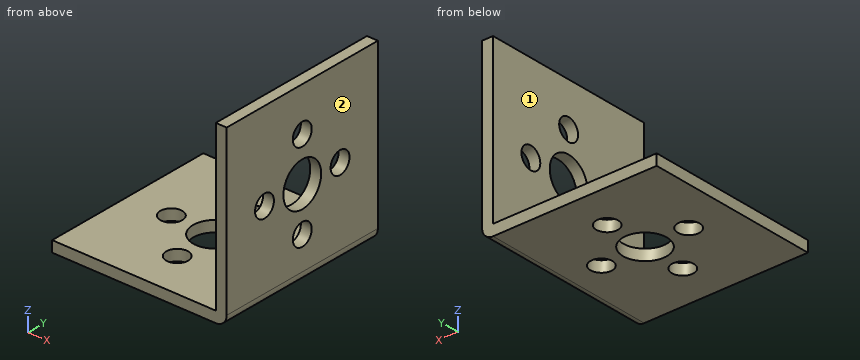
from build123d import *

# Parameters (mm, degrees)
F0_W     = 32
F0_H     = 32
F0_R     = 2
F0_R_2   = 4
F3_DEPTH = 2
F2_W     = 32
F2_H     = 32
F2_R     = 2
F2_R_2   = 4
F4_DEPTH = 2
F5_R     = 2


with BuildPart() as f3:
    # F0 (on Top) → F3 (new body)
    with BuildSketch(Plane.XY):
        Rectangle(F0_W, F0_H)
        with Locations((0, -8)):
            Circle(F0_R, mode=Mode.SUBTRACT)
        with Locations((-8, 0)):
            Circle(F0_R, mode=Mode.SUBTRACT)
        Circle(F0_R_2, mode=Mode.SUBTRACT)
        with Locations((8, 0)):
            Circle(F0_R, mode=Mode.SUBTRACT)
        with Locations((0, 8)):
            Circle(F0_R, mode=Mode.SUBTRACT)
    extrude(amount=F3_DEPTH)

    # F2 (on face) → F4 (join)
    with BuildSketch(Plane(origin=(16, 0, 0), x_dir=(0, -1, 0), z_dir=(-1, 0, 0))):
        with Locations((0, 16)):
            Rectangle(F2_W, F2_H)
        with Locations((0, 8)):
            Circle(F2_R, mode=Mode.SUBTRACT)
        with Locations((-8, 16)):
            Circle(F2_R, mode=Mode.SUBTRACT)
        with Locations((0, 16)):
            Circle(F2_R_2, mode=Mode.SUBTRACT)
        with Locations((8, 16)):
            Circle(F2_R, mode=Mode.SUBTRACT)
        with Locations((0, 24)):
            Circle(F2_R, mode=Mode.SUBTRACT)
    extrude(amount=F4_DEPTH)

    # F5
    f5_edges = [f3.edges().sort_by_distance(p)[0] for p in [
        (16, 0, 0),
    ]]
    fillet(f5_edges, radius=F5_R)


solid = f3.part
The model under review builds one solid part; all positions refer to its coordinate system, in mm. Face numbers are marked on the shaded views. A direction names the side the tool comes from. Give positions to 0.01 mm unless a question says otherwise; leave off trailing zeros. Loops run counter-clockwise (first coordinate to the right, second up) from the corner with the lowest first, then second, coordinate; pieces in that order, holes last. Notation, with made-up numbers: (43.25, 37) -> (94.25, 37) arc R17 ccw to (94.25, 41) -> close; hole circle Ø5 at (-40, -38). An arc over 180 degrees is marked (long way). Write each question's results on one line, items separated by ' | '.
1) Insertion check: pin 1 Ø5 at (x, y) = (8, 0) entering from -Z; pin 2 Ø1.5 at (x, y) = (3, -2) entering from +Z; pin 3 Ø13 at (y, z) = (0, 16) entering from -X. Each pin has a flat end and moves straight along its axis. Give the tip position at first contact, or say it passes through.
Conclusion:
pin 1: stops at z = 0 | pin 2: stops at z = 2 | pin 3: stops at x = 14
2) For line 1 along Y through (x, z) = (0, 0.7); line 2 along Z through (x, y) = (15, 0); line 3 along Z through (x, y) = (5.5, -13), list the stretches that pass through material, from the lowest coordinate up. Write a range as from..to.
Conclusion:
line 1: y = -16..-10, -6..-4, 4..6, 10..16 | line 2: z = 0.27..6, 10..12, 20..22, 26..32 | line 3: z = 0..2
3) Take a section at C-C, the plane z = 8. Give the boundary of the cut face in (x, y), plus the area to 3 significant figures.
Conclusion:
outline: (14, -16) -> (16, -16) -> (16, -2) -> (14, -2) -> close; (14, 2) -> (16, 2) -> (16, 16) -> (14, 16) -> close | area: 56.0 mm^2
4) Take a section at A-A, the plane y = 0. Count the separate pieces of the cut face and the enclosed holes in it, plus the area to 3 significant figures.
Conclusion:
separate pieces: 7 | enclosed holes: 0 | area: 59.1 mm^2
5) Take a section at D-D, the plane y = 8. Give the boundary of the cut face in (x, z), plus the area to 3 significant figures.
Conclusion:
outline: (-16, 0) -> (-2, 0) -> (-2, 2) -> (-16, 2) -> close; (2, 0) -> (14, 0) arc R2 ccw to (16, 2) -> (16, 14) -> (14, 14) -> (14, 2) -> (2, 2) -> close; (14, 18) -> (16, 18) -> (16, 32) -> (14, 32) -> close | area: 107 mm^2
6) Take a section at B-B, the plane x = 8. Give the boundary of the cut face in (y, z).
Conclusion:
outline: (-16, 0) -> (-2, 0) -> (-2, 2) -> (-16, 2) -> close; (2, 0) -> (16, 0) -> (16, 2) -> (2, 2) -> close
7) Tool access review of the marked faces 1 and 2: name each direction out of +Z, -Z, +X, -X, +Y, -Y from which nothing blocks a thin tool from reaching the whole face with its end or side.
Conclusion:
face 1: +Z, -X, +Y, -Y | face 2: +Z, -Z, +X, +Y, -Y
